Could you check a few things on this model? Use its own coordinates, in mm. Coordinates: 2 decimals unless noted, no trailing zeros. Order: outer loops, then holes, each group sorted by start corner. A loop starts at its lowest first (then second) coordinate and runs counter-clockwise, first axis right, second up. Notation, with made-up numbers: (3.25, 38.25) - (37.25, 38.25) arc R22 cw to (37.25, 52.25) - close; hole circle Ø1 at (82, 2). An arc over 180 degrees is marked (long way). One line per item, written item: value.
from build123d import *

# Parameters (mm, degrees)
BOSS_EXTRUDE1_DEPTH = 3.175
SKETCH3_R           = 2.505
CUT_EXTRUDE4_DEPTH  = 4.175


with BuildPart() as part:
    # Sketch1 → Boss-Extrude1 (new body)
    with BuildSketch(Plane.XY):
        with BuildLine():
            Line((-227.394146502, -79.607268705), (-386.144146502, -79.607268705))
            ThreePointArc((-386.144146502, -79.607268705), (-388.389210532, -78.677332735), (-389.319146502, -76.432268705))
            Line((-389.319146502, -76.432268705), (-389.319146502, 120.417731295))
            ThreePointArc((-389.319146502, 120.417731295), (-388.389210532, 122.662795325), (-386.144146502, 123.592731295))
            Line((-386.144146502, 123.592731295), (-227.394146502, 123.592731295))
            ThreePointArc((-227.394146502, 123.592731295), (-225.149082471, 122.662795325), (-224.219146502, 120.417731295))
            Line((-224.219146502, 120.417731295), (-224.219146502, -76.432268705))
            ThreePointArc((-224.219146502, -76.432268705), (-225.149082471, -78.677332735), (-227.394146502, -79.607268705))
        make_face()
        with BuildLine():
            Line((-308.039146502, 118.004731295), (-269.939146502, 118.004731295))
            ThreePointArc((-269.939146502, 118.004731295), (-267.399146502, 115.464731295), (-269.939146502, 112.924731295))
            Line((-269.939146502, 112.924731295), (-308.039146502, 112.924731295))
            ThreePointArc((-308.039146502, 112.924731295), (-310.579146502, 115.464731295), (-308.039146502, 118.004731295))
        make_face(mode=Mode.SUBTRACT)
        with BuildLine():
            Line((-308.039146502, -68.939268705), (-269.939146502, -68.939268705))
            ThreePointArc((-269.939146502, -68.939268705), (-267.399146502, -71.479268705), (-269.939146502, -74.019268705))
            Line((-269.939146502, -74.019268705), (-308.039146502, -74.019268705))
            ThreePointArc((-308.039146502, -74.019268705), (-310.579146502, -71.479268705), (-308.039146502, -68.939268705))
        make_face(mode=Mode.SUBTRACT)
    extrude(amount=BOSS_EXTRUDE1_DEPTH)

    # Sketch3 → Cut-Extrude4 (cut, through all)
    with BuildSketch(Plane.XY.offset(3.175)):
        with Locations((-376.619146502, 110.892731295)):
            Circle(SKETCH3_R)
        with Locations((-376.619146502, -66.907268705)):
            Circle(SKETCH3_R)
        with Locations((-363.919146502, 110.892731295)):
            Circle(SKETCH3_R)
        with Locations((-363.919146502, -66.907268705)):
            Circle(SKETCH3_R)
        with Locations((-351.219146502, 110.892731295)):
            Circle(SKETCH3_R)
        with Locations((-351.219146502, -66.907268705)):
            Circle(SKETCH3_R)
        with Locations((-338.519146502, 110.892731295)):
            Circle(SKETCH3_R)
        with Locations((-338.519146502, -66.907268705)):
            Circle(SKETCH3_R)
        with Locations((-325.819146502, 110.892731295)):
            Circle(SKETCH3_R)
        with Locations((-325.819146502, -66.907268705)):
            Circle(SKETCH3_R)
        with Locations((-313.119146502, 110.892731295)):
            Circle(SKETCH3_R)
        with Locations((-313.119146502, -66.907268705)):
            Circle(SKETCH3_R)
        with Locations((-236.919146502, 110.892731295)):
            Circle(SKETCH3_R)
        with Locations((-236.919146502, -66.907268705)):
            Circle(SKETCH3_R)
        with Locations((-249.619146502, -66.907268705)):
            Circle(SKETCH3_R)
        with Locations((-249.619146502, 110.892731295)):
            Circle(SKETCH3_R)
        with Locations((-262.319146502, -66.907268705)):
            Circle(SKETCH3_R)
        with Locations((-262.319146502, 110.892731295)):
            Circle(SKETCH3_R)
    extrude(amount=-CUT_EXTRUDE4_DEPTH, mode=Mode.SUBTRACT)


solid = part.part
Item 1: Thinking about a two-plate mould opening in Y: for faces 1 (the face through (-365.91, -68.43, 1.61)), 2 (the face through (-340.51, -68.43, 1.61)), 3 (the face through (-306, 23, 3.175)), which applies, pulls with the +Y half, pulls with the -Y half, needs draft (parallel to the pull), parting line crosses it, or undercut?
Conclusion:
face 1: undercut
face 2: undercut
face 3: needs draft
Item 2: If I drill on probe 1 along Y at (x, z) = (-300, 2.5); probe 2 along Y at (x, z) = (-308.5, 2.7), over which ranges is the centre line in solid material (lowest first)?
Conclusion:
probe 1: -79.61 to -74.02, -68.94 to 112.92, 118 to 123.59
probe 2: -79.61 to -73.98, -68.98 to 112.97, 117.96 to 123.59
Item 3: I want a section at B-B on z = 2. Give the number of separate pieces and of enclosed holes in the cut face, then the cut area to 3 significant figures.
Conclusion:
separate pieces: 1
enclosed holes: 20
area: 32,800 mm²
Item 4: I want a section at A-A on x = -304. Please give me the cut outline in (y, z) (3 decimals), then the cut area to 3 significant figures.
Conclusion:
outline: (-79.607, 0) - (-74.019, 0) - (-74.019, 3.175) - (-79.607, 3.175) - close; (-68.939, 0) - (112.925, 0) - (112.925, 3.175) - (-68.939, 3.175) - close; (118.005, 0) - (123.593, 0) - (123.593, 3.175) - (118.005, 3.175) - close
area: 613 mm²
Item 5: I'm going to push a flat-ended pin straight in: pin 1 Ø4.5 at (x, y) = (-236.92, -66.91) entering from +Z. Where does the tip first touch, or does it pass through?
Conclusion:
pin 1: through
